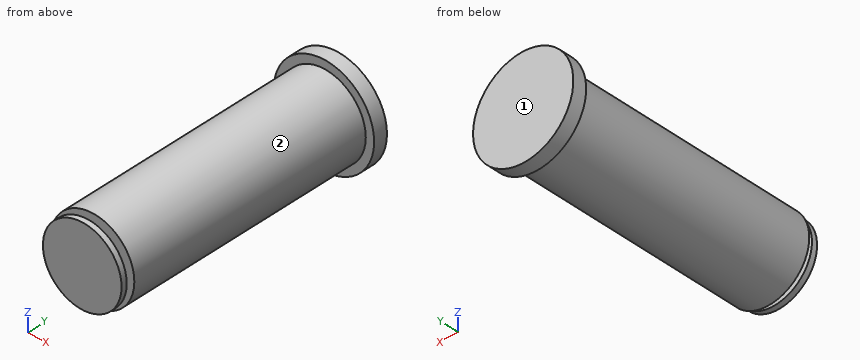
```python
from build123d import *

# Parameters (mm, degrees)
SKETCH1_R           = 15
BOSS_EXTRUDE1_DEPTH = 90
SKETCH2_R           = 18
BOSS_EXTRUDE2_DEPTH = 5
SKETCH3_R           = 2.5
BOSS_EXTRUDE3_DEPTH = 2
SKETCH4_R           = 14.11079173
BOSS_EXTRUDE4_DEPTH = 2


with BuildPart() as part:
    # Sketch1 → Boss-Extrude1 (new body)
    with BuildSketch(Plane(origin=(0, 0, 0), x_dir=(1, 0, 0), z_dir=(0, 1, 0))):
        Circle(SKETCH1_R)
    extrude(amount=BOSS_EXTRUDE1_DEPTH)

    # Sketch2 → Boss-Extrude2 (add)
    with BuildSketch(Plane(origin=(0, 90, 0), x_dir=(1, 0, 0), z_dir=(0, 1, 0))):
        Circle(SKETCH2_R)
    extrude(amount=BOSS_EXTRUDE2_DEPTH)

    # Sketch3 → Boss-Extrude3 (add)
    with BuildSketch(Plane.XZ):
        Circle(SKETCH3_R)
    extrude(amount=BOSS_EXTRUDE3_DEPTH)

    # Sketch4 → Boss-Extrude4 (add)
    with BuildSketch(Plane.XZ.offset(2)):
        Circle(SKETCH4_R)
    extrude(amount=BOSS_EXTRUDE4_DEPTH)


solid = part.part
```
For this review, take the finished solid that the model builds, in its own axes (mm). Face numbers are marked on the shaded views. A direction names the side the tool comes from. Coordinates: 2 decimals unless noted, no trailing zeros. Write each loop counter-clockwise with the first axis right and the second up, starting at its lowest first coordinate (ties: lowest second). Pieces come first, ordered by that corner, then holes.
(1) Add section B-B on x = 9.5. Give the boundary of the cut face in (y, z), then the cut area to 3 significant figures.
(2) Add section A-A on z = 13. Give the boundary of the cut face in (x, y).
(3) Add section D-D on x = 0. Give the boundary of the cut face in (y, z), then the cut area to 3 significant figures.
(4) Tool access review of the marked faces 1 and 2: name each direction out of +Z, -Z, +X, -X, +Y, -Y from which nothing blocks a thin tool from reaching the whole face with its end or side.
(5) For pin 1 Ø12 at (y, z) = (61.5, 13.5) entering from +X; pin 2 Ø1 at (y, z) = (21.5, -13) entering from +X; pin 3 Ø5 at (x, y) = (6, 15) entering from +Z; pin 4 Ø1 at (x, z) = (13, -13.5) entering from -Y, all flat-tipped, find the tip position at first contact; note any pin that passes through.
(6) Wall thickness on probe 1 along Y at (x, z) = (-7, -8); probe 2 along Z at (x, y) = (-0.5, 53); probe 3 along Y at (x, z) = (13, 10): over which ranges is each line inside the solid? List them lowest first.
(7) Add section C-C on z = 0. Give the boundary of the cut face in (x, y), then the cut area to 3 significant figures.
Answer sheet:
1. outline: (-4, -10.43) - (-2, -10.43) - (-2, 10.43) - (-4, 10.43) - close; (0, -11.61) - (90, -11.61) - (90, -15.29) - (95, -15.29) - (95, 15.29) - (90, 15.29) - (90, 11.61) - (0, 11.61) - close
1. area: 2,280 mm2
2. outline: (-12.45, 90) - (-7.48, 90) - (-7.48, 0) - (7.48, 0) - (7.48, 90) - (12.45, 90) - (12.45, 95) - (-12.45, 95) - close; (-5.49, -4) - (5.49, -4) - (5.49, -2) - (-5.49, -2) - close
3. outline: (-4, -14.11) - (-2, -14.11) - (-2, -2.5) - (0, -2.5) - (0, -15) - (90, -15) - (90, -18) - (95, -18) - (95, 18) - (90, 18) - (90, 15) - (0, 15) - (0, 2.5) - (-2, 2.5) - (-2, 14.11) - (-4, 14.11) - close
3. area: 2,950 mm2
4. face 1: +Z, -Z, +X, -X, +Y
4. face 2: -Y
5. pin 1: stops at x = 12.99
5. pin 2: stops at x = 8.29
5. pin 3: stops at z = 14.59
5. pin 4: passes through
6. probe 1: y = -4 to -2, 0 to 95
6. probe 2: z = -14.99 to 14.99
6. probe 3: y = 90 to 95
7. outline: (-18, 90) - (-15, 90) - (-15, 0) - (-2.5, 0) - (-2.5, -2) - (-14.11, -2) - (-14.11, -4) - (14.11, -4) - (14.11, -2) - (2.5, -2) - (2.5, 0) - (15, 0) - (15, 90) - (18, 90) - (18, 95) - (-18, 95) - close
7. area: 2,950 mm2
